The listing builds one solid part. Answer for the finished solid, in the listing's coordinates (mm). A direction names the side the tool comes from. Round coordinates to 2 decimals unless told otherwise and drop trailing zeros. Order: outer loops, then holes, each group sorted by start corner. A loop starts at its lowest first (then second) coordinate and runs counter-clockwise, first axis right, second up. Notation, with made-up numbers: M 18,48 L 57,48 A29 cw 57,83 Z; hole C -26.5,6 d3. An arc over 180 degrees is marked long. Write item = value, one per line. Start each with the question number.
(1) Each of these flat-tipped pins is pushed along its axis until it touches: pin 1 (5 mm diameter, centred on y = 7.5, z = -4, fed in from +X); pin 2 (1 mm diameter, centred on x = -2.5, y = 15.5, fed in from +Z); pin 3 (6 mm diameter, centred on x = -5, y = 23, fed in from +Z). Where does it stop, or does it pass through?
(2) A cutting plane is placed at A-A, the plane y = 27. Determine the outline of the cut face in (x, z).
(3) A cutting plane is placed at B-B, the plane x = 5.75. Determine the outline of the cut face in (y, z).
(4) For a pull along X with two mould halves and no side action, classify faces 1 (the face through (3, 24, -1)), 2 (the face through (-0.7, 0, -1.5)), 3 (the face through (0.921, 7.098, -4.147)), 4 (the face through (2.18, 26.46, -3.84)) as released by +X, released by -X, zero draft, split by the parting line, or undercut.
(5) A cutting plane is placed at C-C, the plane y = 18.5. Determine the outline of the cut face in (x, z).
(6) A cutting plane is placed at D-D, the plane y = 9.75. Determine the outline of the cut face in (x, z), and give its area (3 significant figures).
(7) Straight lines are drawn through the part: probe 1 along Z at (x, y) = (0, 18.75); probe 2 along Y at (x, z) = (-5.25, 2.75). For each, find the intervals that lie inside material, in ascending order. Write a range as from..to.
(8) Which of the six approach directions +Z, -Z, +X, -X, +Y, -Y give full straight-line access (tool end or side, diameter ignored) to faces 5 (the face through (-0.11, 24, 5.22)), 6 (the face through (3, 19, 0)), 7 (the face through (3.4, 29, 3.4))?
Autodesk Inventor part; units mm, degrees
ref_plane "YZ Plane" through (0, 0, 0) normal (1, 0, 0) x (0, 1, 0)
ref_plane "XY Plane" through (0, 0, 0) normal (0, 0, 1) x (1, 0, 0)
sketch "Sketch1" plane through (0, 0, 0) normal (0, 1, 0) x (-1, 0, 0)
  circle A0 centre (0, 0) radius 3.475
  circle A1 centre (0, 0) radius 1.5
  dimension "d0" = 6.95
  dimension "d11" = 3
ref_plane "Work Plane1" through (0, 14, 0) normal (0, 1, 0) x (-1, 0, 0)
sketch "Sketch2" plane through (0, 14, 0) normal (0, 1, 0) x (-1, 0, 0)
  circle A0 centre (0, 0) radius 5
  circle A1 centre (0, 0) radius 3
  dimension "d6" = 10
  dimension "d12" = 6
loft "Loft1" add profiles "Sketch1", "Sketch2" contours A0 | A1 / A0 | A1
extrude "Extrusion2" add sketch "Sketch2" along normal blind 10
hole "Hole3" at (0, 0, 0) direction (0, 1, 0) diameter 3 end through all
loft "Loft2" cut section 1 edges at (0, 0, 1.5) section 2 edges at (3, 14, 0)
sketch "Sketch3" plane through (0, 24, 0) normal (0, 1, 0) x (1, 0, 0)
  circle A0 centre (0, 0) radius 3
  circle A1 centre (0, 0) radius 5.1
  circle A2 centre (0, 0) radius 1.5
  line L0 (0, 5.1) -> (4.4167, 2.55)
  line L1 (4.4167, 2.55) -> (4.4167, -2.55)
  line L2 (4.4167, -2.55) -> (0, -5.1)
  line L3 (0, -5.1) -> (-4.4167, -2.55)
  line L4 (-4.4167, -2.55) -> (-4.4167, 2.55)
  line L5 (-4.4167, 2.55) -> (0, 5.1)
  circle A3 centre (0, 0) radius 8
  dimension "d43" = 10.2
  dimension "d42" = 6
  dimension "d44" = 16
extrude "Extrusion3" add sketch "Sketch3" along normal blind 5 contours A1 L1 | L0 A1 | A1 L2 | L5 A1 | A1 L3 | L4 A1 | A3
properties part number "vacuum-nozzle-shaft"
Reported:
q1.pin_1 = 4.06
q1.pin_2 = 4.58
q1.pin_3 = 7.7
q2.outline = C 0,0 d16; hole M -4.42,-2.55 L 0,-5.1 L 4.42,-2.55 L 4.42,2.55 L 0,5.1 L -4.42,2.55 Z
q3.outline = M 24,-5.56 L 29,-5.56 L 29,5.56 L 24,5.56 Z
q4.face_1 = undercut
q4.face_2 = zero draft
q4.face_3 = split by the parting line
q4.face_4 = undercut
q5.outline = C 0,0 d10; hole C 0,0 d6
q6.outline = C 0,0 d9.07; hole C 0,0 d5.09
q6.area = 44.3 mm²
q7.probe_1 = -5..-3, 3..5
q7.probe_2 = 24..29
q8.face_5 = -Y
q8.face_6 = +Y
q8.face_7 = +Z, -Z, +X, -X, +Y
